```python
from build123d import *

# Parameters (mm, degrees)
F1_DEPTH = 228.6
F3_D     = 23.876


with BuildPart() as f1:
    # F0 (on Front) → F1 (new body, symmetric)
    with BuildSketch(Plane.XZ):
        with BuildLine():
            Line((6.3500000013, 88.9), (0, 88.9))
            Line((0, 88.9), (0, 0))
            Line((0, 0), (127, 0))
            Line((127, 0), (127, 6.35))
            ThreePointArc((127, 6.35), (125.1401280605, 10.8401280605), (120.65, 12.7))
            Line((120.65, 12.7), (23.8125000013, 12.7))
            ThreePointArc((23.8125000013, 12.7), (15.9547758954, 15.9547758941), (12.7000000013, 23.8125))
            Line((12.7000000013, 23.8125), (12.7000000013, 82.55))
            ThreePointArc((12.7000000013, 82.55), (10.8401280618, 87.0401280605), (6.3500000013, 88.9))
        make_face()
    extrude(amount=F1_DEPTH, both=True)

    # F3 (through all)
    with Locations(Plane(origin=(0, 0, 0), x_dir=(0, 1, 0), z_dir=(-1, 0, 0))):
        with Locations((-152.4, -50.8), (0, -50.8), (152.4, -50.8)):
            Hole(F3_D / 2)


solid = f1.part
```
Source: CAD feature listing. Evaluate the final solid. Frame: model axes, mm. A direction names the side the tool comes from. Round coordinates to 2 decimals unless told otherwise and drop trailing zeros. Order: outer loops, then holes, each group sorted by start corner. A loop starts at its lowest first (then second) coordinate and runs counter-clockwise, first axis right, second up. Notation, with made-up numbers: (9.25, 66.5) -> (35.25, 66.5) arc R37 cw to (35.25, 104.5) -> close; hole circle Ø7 at (78, 89.5). An arc over 180 degrees is marked (long way). Use CSV: the item, a comma, the result in double quotes.
(1) Section B-B on z = 43.5. Return the cut outline in (x, y).
Report:
outline,"(0, -228.6) -> (12.7, -228.6) -> (12.7, -161.85) -> (0, -161.85) -> close; (0, -142.95) -> (12.7, -142.95) -> (12.7, -9.45) -> (0, -9.45) -> close; (0, 9.45) -> (12.7, 9.45) -> (12.7, 142.95) -> (0, 142.95) -> close; (0, 161.85) -> (12.7, 161.85) -> (12.7, 228.6) -> (0, 228.6) -> close"
(2) Section D-D on x = 42. Return the cut outline in (y, z), and give its area (3 significant figures).
Report:
outline,"(-228.6, 0) -> (228.6, 0) -> (228.6, 12.7) -> (-228.6, 12.7) -> close"
area,"5,810 mm^2"
(3) Pull-direction query (Z, two-part tool) for faces 3 (the face through (40, -228.6, 12)), 4 (the face through (6.439, 1.554, 38.964)), 5 (the face through (16.04, -3.2, 15.87)); classes: +Z half, -Z half, draft (parallel to the pull), parting line (faces both ways), or undercut.
Report:
face 3,"draft"
face 4,"undercut"
face 5,"+Z half"
(4) Access query for faces 1 (the face through (12.7, -3, 66)), 2 (the face through (6.439, -163.787, 47.214)). Directions: +Z, -Z, +X, -X, +Y, -Y. A direction counts if a zero-diameter tool reaches every point of the face in a straight line with its end or side. Return the directions, or none.
Report:
face 1,"+Z, +X, +Y, -Y"
face 2,"+X, -X"
(5) First-contact query: pin 1 Ø5 at (x, y) = (46.5, 45.5) entering from +Z. Flat tip, straight axial feed; report the tip coordinate or a pass-through.
Report:
pin 1,"z = 12.7"
(6) Ray query, L1, parallel to Y at x = 7.25, z = 50.8; L2, parallel to Z at x = 29.5, y = 174. Return the intervals inside material, ascending.
Report:
L1,"-228.6 to -164.34, -140.46 to -11.94, 11.94 to 140.46, 164.34 to 228.6"
L2,"0 to 12.7"
